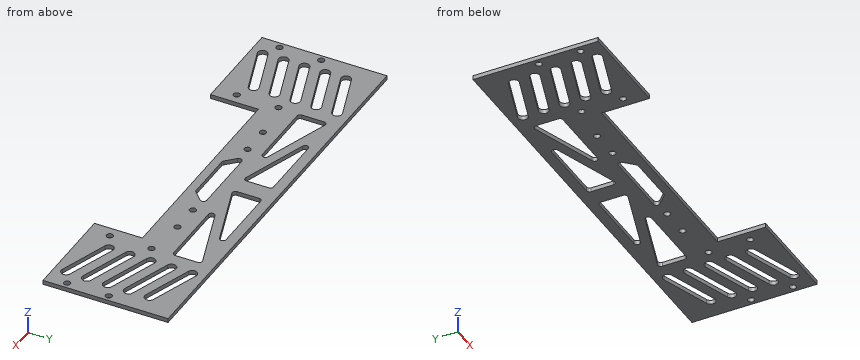
```python
from build123d import *

# Parameters (mm, degrees)
SKETCH_1_R      = 1.55
EXTRUDE_1_DEPTH = 2


with BuildPart() as part:
    # 草图1 → 凸台-拉伸1 (new body)
    with BuildSketch(Plane.XY):
        Polygon((69.118055556, 5.822916667), (69.118055556, -30.177083333), (22.118055556, -30.177083333), (22.118055556, -7.177083333), (-83.881944444, -7.177083333), (-83.881944444, -30.177083333), (-130.881944444, -30.177083333), (-130.881944444, 5.822916667), (-130.881944444, 29.822916667), (69.118055556, 29.822916667), align=None)
        with Locations((-127.881944444, -0.177083333)):
            Circle(SKETCH_1_R, mode=Mode.SUBTRACT)
        with Locations((-127.881944444, -20.177083333)):
            Circle(SKETCH_1_R, mode=Mode.SUBTRACT)
        with Locations((-88.881944444, -0.177083333)):
            Circle(SKETCH_1_R, mode=Mode.SUBTRACT)
        with Locations((-88.881944444, -20.177083333)):
            Circle(SKETCH_1_R, mode=Mode.SUBTRACT)
        with Locations((27.118055556, -0.177083333)):
            Circle(SKETCH_1_R, mode=Mode.SUBTRACT)
        with Locations((27.118055556, -20.177083333)):
            Circle(SKETCH_1_R, mode=Mode.SUBTRACT)
        with Locations((66.118055556, -0.177083333)):
            Circle(SKETCH_1_R, mode=Mode.SUBTRACT)
        with Locations((66.118055556, -20.177083333)):
            Circle(SKETCH_1_R, mode=Mode.SUBTRACT)
        with Locations((-69.881944444, 2.322916667)):
            Circle(SKETCH_1_R, mode=Mode.SUBTRACT)
        with Locations((-55.881944444, 2.322916667)):
            Circle(SKETCH_1_R, mode=Mode.SUBTRACT)
        with Locations((-5.881944444, 2.322916667)):
            Circle(SKETCH_1_R, mode=Mode.SUBTRACT)
        with Locations((8.118055556, 2.322916667)):
            Circle(SKETCH_1_R, mode=Mode.SUBTRACT)
        with BuildLine():
            Line((-96.308316621, 21.419007892), (-119.878819488, 13.358099985))
            ThreePointArc((-119.878819488, 13.358099985), (-122.854752457, 14.817267118), (-121.395585324, 17.793200088))
            Line((-121.395585324, 17.793200088), (-97.825082457, 25.854107995))
            ThreePointArc((-97.825082457, 25.854107995), (-94.849149487, 24.394940861), (-96.308316621, 21.419007892))
        make_face(mode=Mode.SUBTRACT)
        with BuildLine():
            Line((-96.308316621, 11.419007892), (-119.878819488, 3.358099985))
            ThreePointArc((-119.878819488, 3.358099985), (-122.854752457, 4.817267118), (-121.395585324, 7.793200088))
            Line((-121.395585324, 7.793200088), (-97.825082457, 15.854107995))
            ThreePointArc((-97.825082457, 15.854107995), (-94.849149487, 14.394940861), (-96.308316621, 11.419007892))
        make_face(mode=Mode.SUBTRACT)
        with BuildLine():
            Line((-96.308316621, 1.419007892), (-119.878819488, -6.641900015))
            ThreePointArc((-119.878819488, -6.641900015), (-122.854752457, -5.182732882), (-121.395585324, -2.206799912))
            Line((-121.395585324, -2.206799912), (-97.825082457, 5.854107995))
            ThreePointArc((-97.825082457, 5.854107995), (-94.849149487, 4.394940861), (-96.308316621, 1.419007892))
        make_face(mode=Mode.SUBTRACT)
        with BuildLine():
            Line((-96.308316621, -8.580992108), (-119.878819488, -16.641900015))
            ThreePointArc((-119.878819488, -16.641900015), (-122.854752457, -15.182732882), (-121.395585324, -12.206799912))
            Line((-121.395585324, -12.206799912), (-97.825082457, -4.145892005))
            ThreePointArc((-97.825082457, -4.145892005), (-94.849149487, -5.605059139), (-96.308316621, -8.580992108))
        make_face(mode=Mode.SUBTRACT)
        with BuildLine():
            Line((-96.308316621, -18.580992108), (-119.878819488, -26.641900015))
            ThreePointArc((-119.878819488, -26.641900015), (-122.854752457, -25.182732882), (-121.395585324, -22.206799912))
            Line((-121.395585324, -22.206799912), (-97.825082457, -14.145892005))
            ThreePointArc((-97.825082457, -14.145892005), (-94.849149487, -15.605059139), (-96.308316621, -18.580992108))
        make_face(mode=Mode.SUBTRACT)
        with BuildLine():
            Line((34.544427732, -18.580992108), (58.114930599, -26.641900015))
            ThreePointArc((58.114930599, -26.641900015), (61.090863569, -25.182732882), (59.631696435, -22.206799912))
            Line((59.631696435, -22.206799912), (36.061193568, -14.145892005))
            ThreePointArc((36.061193568, -14.145892005), (33.085260599, -15.605059139), (34.544427732, -18.580992108))
        make_face(mode=Mode.SUBTRACT)
        with BuildLine():
            Line((34.544427732, -8.580992108), (58.114930599, -16.641900015))
            ThreePointArc((58.114930599, -16.641900015), (61.090863569, -15.182732882), (59.631696435, -12.206799912))
            Line((59.631696435, -12.206799912), (36.061193568, -4.145892005))
            ThreePointArc((36.061193568, -4.145892005), (33.085260599, -5.605059139), (34.544427732, -8.580992108))
        make_face(mode=Mode.SUBTRACT)
        with BuildLine():
            Line((34.544427732, 1.419007892), (58.114930599, -6.641900015))
            ThreePointArc((58.114930599, -6.641900015), (61.090863569, -5.182732882), (59.631696435, -2.206799912))
            Line((59.631696435, -2.206799912), (36.061193568, 5.854107995))
            ThreePointArc((36.061193568, 5.854107995), (33.085260599, 4.394940861), (34.544427732, 1.419007892))
        make_face(mode=Mode.SUBTRACT)
        with BuildLine():
            Line((34.544427732, 11.419007892), (58.114930599, 3.358099985))
            ThreePointArc((58.114930599, 3.358099985), (61.090863569, 4.817267118), (59.631696435, 7.793200088))
            Line((59.631696435, 7.793200088), (36.061193568, 15.854107995))
            ThreePointArc((36.061193568, 15.854107995), (33.085260599, 14.394940861), (34.544427732, 11.419007892))
        make_face(mode=Mode.SUBTRACT)
        with BuildLine():
            Line((34.544427732, 21.419007892), (58.114930599, 13.358099985))
            ThreePointArc((58.114930599, 13.358099985), (61.090863569, 14.817267118), (59.631696435, 17.793200088))
            Line((59.631696435, 17.793200088), (36.061193568, 25.854107995))
            ThreePointArc((36.061193568, 25.854107995), (33.085260599, 24.394940861), (34.544427732, 21.419007892))
        make_face(mode=Mode.SUBTRACT)
        with BuildLine():
            Line((-86.707081272, 23.202972479), (-55.025491003, 12.527575239))
            ThreePointArc((-55.025491003, 12.527575239), (-54.024230917, 10.863417849), (-55.504468546, 9.60610399))
            Line((-55.504468546, 9.60610399), (-87.186058815, 9.60610399))
            ThreePointArc((-87.186058815, 9.60610399), (-88.246718986, 10.045443818), (-88.686058815, 11.10610399))
            Line((-88.686058815, 11.10610399), (-88.686058815, 21.781501229))
            ThreePointArc((-88.686058815, 21.781501229), (-88.061139864, 22.99979231), (-86.707081272, 23.202972479))
        make_face(mode=Mode.SUBTRACT)
        with BuildLine():
            Line((-68.415657461, 24.859225404), (-36.734067193, 24.859225404))
            ThreePointArc((-36.734067193, 24.859225404), (-35.673407021, 24.419885576), (-35.234067193, 23.359225404))
            Line((-35.234067193, 23.359225404), (-35.234067193, 12.683828165))
            ThreePointArc((-35.234067193, 12.683828165), (-35.858986143, 11.465537084), (-37.213044735, 11.262356915))
            Line((-37.213044735, 11.262356915), (-68.894635004, 21.937754155))
            ThreePointArc((-68.894635004, 21.937754155), (-69.89589509, 23.601911545), (-68.415657461, 24.859225404))
        make_face(mode=Mode.SUBTRACT)
        with BuildLine():
            Line((26.922169926, 21.781501229), (26.922169926, 11.10610399))
            ThreePointArc((26.922169926, 11.10610399), (26.482830097, 10.045443818), (25.422169926, 9.60610399))
            Line((25.422169926, 9.60610399), (-6.259420343, 9.60610399))
            ThreePointArc((-6.259420343, 9.60610399), (-7.739657972, 10.863417849), (-6.738397886, 12.527575239))
            Line((-6.738397886, 12.527575239), (24.943192383, 23.202972479))
            ThreePointArc((24.943192383, 23.202972479), (26.297250975, 22.99979231), (26.922169926, 21.781501229))
        make_face(mode=Mode.SUBTRACT)
        with BuildLine():
            Line((7.130746115, 21.937754155), (-24.550844154, 11.262356915))
            ThreePointArc((-24.550844154, 11.262356915), (-25.904902746, 11.465537084), (-26.529821696, 12.683828165))
            Line((-26.529821696, 12.683828165), (-26.529821696, 23.359225404))
            ThreePointArc((-26.529821696, 23.359225404), (-26.090481868, 24.419885576), (-25.029821696, 24.859225404))
            Line((-25.029821696, 24.859225404), (6.651768572, 24.859225404))
            ThreePointArc((6.651768572, 24.859225404), (8.132006201, 23.601911545), (7.130746115, 21.937754155))
        make_face(mode=Mode.SUBTRACT)
        with BuildLine():
            Line((-14.846833492, 4.237725323), (-46.917055397, 4.237725323))
            ThreePointArc((-46.917055397, 4.237725323), (-48.302874696, 3.311750471), (-47.977715569, 1.677065151))
            Line((-47.977715569, 1.677065151), (-43.630536244, -2.670114174))
            ThreePointArc((-43.630536244, -2.670114174), (-43.14390122, -2.995273301), (-42.569876072, -3.109454002))
            Line((-42.569876072, -3.109454002), (-19.194012817, -3.109454002))
            ThreePointArc((-19.194012817, -3.109454002), (-18.619987668, -2.995273301), (-18.133352645, -2.670114174))
            Line((-18.133352645, -2.670114174), (-13.78617332, 1.677065151))
            ThreePointArc((-13.78617332, 1.677065151), (-13.461014193, 3.311750471), (-14.846833492, 4.237725323))
        make_face(mode=Mode.SUBTRACT)
    extrude(amount=EXTRUDE_1_DEPTH)


solid = part.part
```
Design review of the part built by this model. Coordinates are the model's own, in mm. Round coordinates to 2 decimals unless told otherwise and drop trailing zeros. Write each loop counter-clockwise with the first axis right and the second up, starting at its lowest first coordinate (ties: lowest second). Pieces come first, ordered by that corner, then holes.
Item 1: Clearance check with a flat-ended pin moving along its axis: pin 1 Ø0.6 at (x, z) = (-52.5, 1) entering from -Y. State where the tip first meets the part, or that it passes through.
Item 2: We need section C-C on z = 1.55. State how many separate pieces and enclosed holes the cut face has, and give its area (3 significant figures).
Item 3: For probe 1 along Y at (x, z) = (-97, 1.3); probe 2 along Y at (x, z) = (-99, 0.75); probe 3 along Y at (x, z) = (-55.5, 0.3), list the stretches that pass through material, from the lowest coordinate up.
Item 4: We need section B-B on x = 48. Write out the cut boundary in (y, z), and give its area (3 significant figures).
Item 5: We need section A-A on x = -31. Write out the cut boundary in (y, z).
Returned:
1. pin 1: stops at y = -7.18
2. separate pieces: 1
2. enclosed holes: 27
2. area: 6,740 mm2
3. probe 1: y = -30.18 to -18.82, -14.02 to -8.82, -4.02 to 1.18, 5.98 to 11.18, 15.98 to 21.18, 25.98 to 29.82
3. probe 2: y = -30.18 to -19.5, -14.55 to -9.5, -4.55 to 0.5, 5.45 to 10.5, 15.45 to 20.5, 25.45 to 29.82
3. probe 3: y = -7.18 to 0.82, 3.83 to 9.61, 12.69 to 17.42, 24.86 to 29.82
4. outline: (-30.18, 0) - (-23.18, 0) - (-23.18, 2) - (-30.18, 2) - close; (-18.23, 0) - (-13.18, 0) - (-13.18, 2) - (-18.23, 2) - close; (-8.23, 0) - (-3.18, 0) - (-3.18, 2) - (-8.23, 2) - close; (1.77, 0) - (6.82, 0) - (6.82, 2) - (1.77, 2) - close; (11.77, 0) - (16.82, 0) - (16.82, 2) - (11.77, 2) - close; (21.77, 0) - (29.82, 0) - (29.82, 2) - (21.77, 2) - close
4. area: 70.5 mm2
5. outline: (-7.18, 0) - (-3.11, 0) - (-3.11, 2) - (-7.18, 2) - close; (4.24, 0) - (29.82, 0) - (29.82, 2) - (4.24, 2) - close
